Autodesk Inventor part; units mm, degrees
ref_plane "Work Plane1" through (-14.5, 14, -2) normal (-1, 0, 0) x (0, 0, -1)
ref_plane "YZ Plane" through (0, 0, 0) normal (1, 0, 0) x (0, 1, 0)
ref_plane "XZ Plane" through (0, 0, 0) normal (0, 1, 0) x (-1, 0, 0)
sketch "Sketch1" plane through (0, 0, 0) normal (0, 1, 0) x (-1, 0, 0)
  line L0 (0, 0) -> (200, 0)
  line L1 (200, 0) -> (200, -150)
  line L2 (200, -150) -> (0, -150)
  line L3 (0, -150) -> (0, 0)
  dimension "d0" = 200
  dimension "d1" = 150
extrude "Extrusion1" add sketch "Sketch1" along normal blind 2
sketch "Sketch2" plane through (0, 2, 0) normal (0, 1, 0) x (1, 0, 0)
  line L0 (-200, 0) -> (0, 0)
  line L1 (-200, 0) -> (-200, 2)
  line L2 (-200, 150) -> (-200, 0)
  line L3 (-200, 2) -> (-2, 2)
  line L4 (-2, 2) -> (-2, 150)
  line L5 (0, 150) -> (-200, 150)
  line L6 (-200, 2) -> (-200, 150)
  line L7 (-200, 150) -> (-2, 150)
  dimension "d4" = 2
  dimension "d5" = 198
extrude "Extrusion2" add sketch "Sketch2" along normal blind 2
sketch "Sketch3" plane through (0, 4, 0) normal (0, 1, 0) x (1, 0, 0)
  line L0 (0, 0) -> (0, 150)
  line L1 (0, 0) -> (-198, 0)
  line L2 (-198, 0) -> (-198, 148)
  line L3 (-198, 148) -> (0, 148)
  line L4 (0, 148) -> (0, 0)
  line L5 (0, 150) -> (-200, 150)
  line L6 (-200, 150) -> (0, 150)
  line L7 (0, 150) -> (0, 0)
  line L8 (0, 0) -> (-200, 0)
  line L9 (-200, 0) -> (-200, 150)
  dimension "d8" = 198
  dimension "d9" = 148
extrude "Extrusion3" add sketch "Sketch3" along normal blind 100 and the other way blind 2 contours L3 L2 L8 L9 L5 L0
sketch "Sketch4" plane through (0, 4, 0) normal (0, 1, 0) x (1, 0, 0)
  line L0 (-198, 2) -> (-2, 2)
  line L1 (-198, 2) -> (-196, 2)
  line L2 (-196, 2) -> (-196, 146)
  line L3 (-2, 148) -> (-198, 148)
  line L4 (-196, 146) -> (-2, 146)
  line L5 (-2, 2) -> (-2, 148)
  line L6 (-2, 2) -> (-198, 2)
  line L7 (-198, 2) -> (-198, 148)
  line L8 (-198, 148) -> (-2, 148)
  line L9 (-2, 148) -> (-2, 2)
  point P0 (0, 0)
  dimension "d14" = 2
  dimension "d15" = 144
extrude "Extrusion4" add sketch "Sketch4" along normal blind 100 contours L7 L3 L5 L4 L2 L0
sketch "Sketch7" plane through (0, 4, 0) normal (0, 1, 0) x (1, 0, 0)
  line L0 (-196, 2) -> (-2, 2)
  line L1 (-196, 2) -> (-196, 3)
  line L2 (-196, 146) -> (-196, 2)
  line L3 (-196, 3) -> (-191, 3)
  line L4 (-191, 3) -> (-191, 8)
  line L5 (-191, 8) -> (-196, 8)
  point P0 (0, 0)
  point P1 (-196, 117.9293)
  dimension "d36" = 1
  dimension "d37" = 5
  dimension "d38" = 5
extrude "Extrusion7" add sketch "Sketch7" along normal blind 5
fillet "Fillet2" radius 2.5 1 edges at (-191, 9, -5.5)
sketch "Sketch9" plane through (0, 4, 0) normal (0, 1, 0) x (1, 0, 0)
  line L0 (-196, 2) -> (-2, 2)
  line L1 (-2, 2) -> (-2, 3)
  line L2 (-2, 2) -> (-2, 146)
  line L3 (-2, 3) -> (-3, 3)
  line L4 (-3, 3) -> (-8, 3)
  line L5 (-8, 3) -> (-8, 8)
  line L6 (-8, 8) -> (-3, 8)
  line L7 (-3, 8) -> (-3, 3)
  point P0 (0, 0)
  dimension "d45" = 1
  dimension "d46" = 1
  dimension "d47" = 5
  dimension "d48" = 5
extrude "Extrusion9" add sketch "Sketch9" along normal blind 5
fillet "Fillet3" radius 2.5 2 edges at (-8, 9, -5.5) (-3, 9, -5.5)
sketch "Sketch10" plane through (-8, 4, -3) normal (0, 0, 1) x (1, 0, 0)
  arc A0 (5, 2.5) -> (0, 2.5) centre (2.5, 2.5) ccw
  circle A1 centre (2.5, 2.5) radius 1
  point P0 (8, -4)
  dimension "d52" = 2
extrude "Extrusion10" cut sketch "Sketch10" against normal blind 5
sketch "Sketch11" plane through (0, 4, 0) normal (0, 1, 0) x (1, 0, 0)
  line L0 (-2, 146) -> (-196, 146)
  line L1 (-2, 146) -> (-3, 146)
  line L2 (-3, 146) -> (-8, 146)
  line L3 (-8, 146) -> (-8, 141)
  line L4 (-8, 141) -> (-3, 141)
  line L5 (-3, 141) -> (-3, 146)
  point P0 (0, 0)
  point P1 (-144.9293, 146)
  dimension "d55" = 1
  dimension "d56" = 5
  dimension "d57" = 5
extrude "Extrusion11" add sketch "Sketch11" along normal blind 5
fillet "Fillet4" radius 2.5 1 edges at (-5.5, 9, -141)
sketch "Sketch12" plane through (-3, 4, -141) normal (1, 0, 0) x (0, 0, -1)
  arc A0 (2.5, 5) -> (0, 2.5) centre (2.5, 2.5) ccw
  circle A1 centre (2.5, 2.5) radius 1
  point P0 (-141, -4)
  dimension "d61" = 2
extrude "Extrusion12" cut sketch "Sketch12" against normal blind 5
sketch "Sketch13" plane through (-196, 104, -146) normal (0, 0, 1) x (1, 0, 0)
  line L0 (0, 0) -> (194, 0)
  line L1 (194, 0) -> (193, 0)
  line L2 (193, 0) -> (193, -1)
  line L3 (193, -1) -> (188, -1)
  line L4 (188, -1) -> (188, -6)
  line L5 (188, -6) -> (193, -6)
  line L6 (193, -6) -> (193, -1)
  point P0 (196, -104)
  dimension "d64" = 1
  dimension "d65" = 1
  dimension "d66" = 5
  dimension "d67" = 5
extrude "Extrusion13" add sketch "Sketch13" along normal blind 5
fillet "Fillet5" radius 2.5 2 edges at (-5.5, 103, -141) (-5.5, 98, -141)
sketch "Sketch14" plane through (-3, 98, -146) normal (1, 0, 0) x (0, 0, -1)
  arc A0 (-2.5, 5) -> (-2.5, 0) centre (-2.5, 2.5) ccw
  circle A1 centre (-2.5, 2.5) radius 1
  point P0 (-146, -98)
  dimension "d71" = 2
extrude "Extrusion14" cut sketch "Sketch14" against normal blind 5
sketch "Sketch15" plane through (-196, 4, -2) normal (1, 0, 0) x (0, 0, -1)
  line L0 (0, 100) -> (0, -2)
  line L1 (0, 100) -> (1, 100)
  line L2 (148, 100) -> (-2, 100)
  line L3 (1, 100) -> (1, 99)
  line L4 (1, 99) -> (6, 99)
  line L5 (6, 99) -> (6, 94)
  line L6 (6, 94) -> (1, 94)
  line L7 (1, 94) -> (1, 99)
  point P0 (-2, -4)
  dimension "d74" = 1
  dimension "d75" = 1
  dimension "d76" = 5
  dimension "d77" = 5
extrude "Extrusion15" add sketch "Sketch15" along normal blind 5
fillet "Fillet6" radius 2.5 2 edges at (-191, 103, -5.5) (-191, 98, -5.5)
sketch "Sketch17" plane through (0, 4, 0) normal (0, 1, 0) x (1, 0, 0)
  point P0 (0, 0)
sketch "Sketch18" plane through (0, 4, 0) normal (0, 1, 0) x (1, 0, 0)
  line L0 (-196, 2) -> (-196, 146)
  line L1 (-196, 84.7457) -> (-26, 84.7457)
  line L2 (0, 0) -> (0, 150)
  line L3 (-26, 84.7457) -> (-26, 146)
  line L4 (-196, 146) -> (-2, 146)
  line L5 (-26, 84.7457) -> (-26, 2)
  line L6 (-196, 2) -> (-2, 2)
  line L7 (-26, 143.5) -> (-27, 143.5)
  line L8 (-27, 143.5) -> (-2, 143.5)
  line L9 (-2, 148) -> (-2, 2)
  line L10 (-14.5, 143.5) -> (-14.5, 2)
  line L11 (-14.5, 143.5) -> (-16.2266, 143.5)
  line L12 (-16.2266, 143.5) -> (-16.2266, 2)
  line L13 (-16.2266, 2) -> (-14.5, 2)
  line L14 (-14.5, 2) -> (-14.5, 143.5)
  line L15 (-16.2266, 143.5) -> (-14.5, 143.5)
  line L16 (-14.5, 143.5) -> (-14.5, 2)
  line L17 (-14.5, 2) -> (-16.2266, 2)
  line L18 (-16.2266, 2) -> (-16.2266, 143.5)
  dimension "d84" = 170
  dimension "d85" = 1
sketch "Sketch19" plane through (0, 4, 0) normal (0, 1, 0) x (1, 0, 0)
  point P0 (0, 0)
extrude "Extrusion17" add sketch "Sketch18" along normal blind 10 contours L12 L8 L10 L6
ref_plane "Work Plane1" through (-14.5, 14, -2) normal (-1, 0, 0) x (0, 0, -1)
mirror "Mirror1" about plane through (-14.5, 4, -2) normal (1, 0, 0) of "Fillet3", "Extrusion9", "Extrusion11", "Fillet4"
sketch "Sketch20" plane through (0, 2, 0) normal (0, 1, 0) x (1, 0, 0)
  line L0 (-26, 143.5) -> (-21, 143.5)
  line L1 (-21, 143.5) -> (-20, 143.5)
  line L2 (-8, 146) -> (-21, 146)
  line L3 (-2, 148) -> (-2, 2)
  line L4 (-20, 146) -> (-2, 146)
  line L5 (-2, 146) -> (-2, 2)
  line L6 (-2, 2) -> (-20, 2)
  line L7 (-20, 2) -> (-20, 146)
  line L8 (0, 148) -> (-2, 148)
  line L9 (-20, 2) -> (-2, 2)
  line L10 (-2, 2) -> (-2, 148)
  line L11 (-2, 148) -> (-20, 148)
  line L12 (-20, 148) -> (-20, 2)
  point P0 (0, 0)
  dimension "d88" = 1
extrude "Extrusion18" cut sketch "Sketch20" along normal blind 1000
sketch "Sketch21" plane through (0, 2, 0) normal (0, 1, 0) x (1, 0, 0)
  line L0 (-20, 148) -> (-20, 2)
  line L1 (-20, 2) -> (-18, 2)
  line L2 (-198, 0) -> (0, 0)
  line L3 (0, 150) -> (-200, 150)
  line L4 (-18, 0) -> (0, 0)
  line L5 (0, 0) -> (0, 150)
  line L6 (0, 150) -> (-18, 150)
  line L7 (-18, 150) -> (-18, 0)
  dimension "d91" = 2
extrude "Extrusion19" cut sketch "Sketch21" along normal mid plane 1000
sketch "Sketch23" plane through (0, 4, 0) normal (0, 1, 0) x (1, 0, 0)
  point P0 (0, 0)
properties part number "kevnat part1"
Build history of the part. All positions in model axes, mm. A direction names the side the tool comes from. Round coordinates to 2 decimals unless told otherwise and drop trailing zeros. Loops run counter-clockwise (first coordinate to the right, second up) from the corner with the lowest first, then second, coordinate; pieces in that order, holes last.
Item 1: Drill centre lines: line 1 along Z through (x, y) = (-170.5, 64.5); line 2 along X through (y, z) = (68, -11); line 3 along Y through (x, z) = (-59.5, -9). Where is each one in solid material? Low to high.
Item 2: Saw through at C-C (x = -41.5). List the corners of the cut face in (y, z).
Item 3: Pin check, flat tips, straight feed: P1, Ø1.5, axis at x = -106.5, y = 13.5, coming from the +Z side; P2, Ø0.8, axis at y = 5.5, z = -5, coming from the +X side; P3, Ø4, axis at x = -23, y = 6.5, coming from the +Z side. Stop position of each tip, or through.
Item 4: Saw through at B-B (y = 28). List the corners of the cut face in (x, z), then the cut area to 3 significant figures.
Item 5: Which spindle directions (+Z, -Z, +X, -X, +Y, -Y) get a long thin tool onto all of the face, cutting with end or side? Do faces 1 (the face through (-108.6, 1.7, 0)), 2 (the face through (-109.4, 3.7, -2)), 3 (the face through (-26, 6, -144)), 4 (the face through (-200, 51, -74)), 5 (the face through (-24, 6, -8)). Say none if no direction does.
Item 6: Saw through at A-A (z = -97.5). List the corners of the cut face in (x, y).
Item 7: Two-plate mould, pull along Z, no slides. Class faces 6 (the face through (-18, 1.7, -75.4)), 7 (the face through (-194, 101, -8)), 8 (the face through (-193, 6, -8)), 9 (the face through (-23, 6, -3)): released by +Z, released by -Z, zero draft, split by the parting line, or undercut.
Worked answers:
1. line 1: z = -150 to -146
1. line 2: x = -200 to -196
1. line 3: y = 0 to 4
2. outline: (0, -150) - (104, -150) - (104, -146) - (4, -146) - (4, -2) - (2, -2) - (2, 0) - (0, 0) - close
3. P1: stops at z = -146
3. P2: stops at x = -21
3. P3: stops at z = -3
4. outline: (-200, -150) - (-18, -150) - (-18, -148) - (-20, -148) - (-20, -146) - (-196, -146) - (-196, -2) - (-198, -2) - (-198, 0) - (-200, 0) - close
4. area: 1,300 mm2
5. face 1: +Z, +X, -X, +Y, -Y
5. face 2: +Z, +X, +Y
5. face 3: +Z, +Y
5. face 4: +Z, -Z, -X, +Y, -Y
5. face 5: +X, +Y
6. outline: (-200, 0) - (-18, 0) - (-18, 2) - (-20, 2) - (-20, 4) - (-196, 4) - (-196, 104) - (-200, 104) - close
7. face 6: zero draft
7. face 7: undercut
7. face 8: undercut
7. face 9: released by +Z
